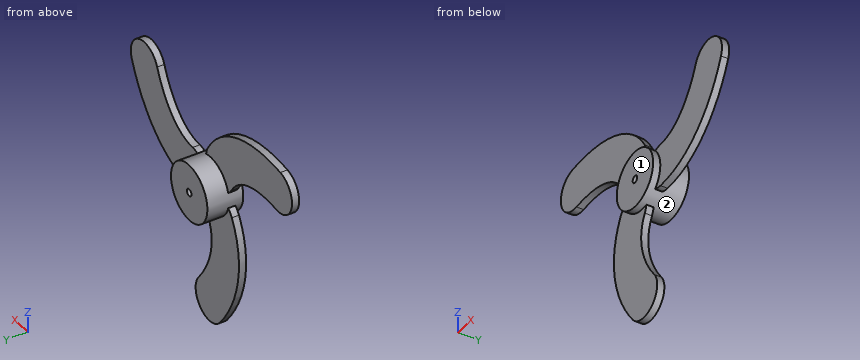
```python
from build123d import *

# Parameters (mm, degrees)
SKETCH1_R               = 4
BOSS_EXTRUDE1_DEPTH     = 5
BOSS_EXTRUDE2_START     = 1
BOSS_EXTRUDE2_DEPTH     = 1
SKETCH3_R               = 0.5
CUT_EXTRUDE1_DEPTH      = 1
CUT_EXTRUDE1_DEPTH_BACK = 6


with BuildPart() as part:
    # Sketch1 → Boss-Extrude1 (new body)
    with BuildSketch(Plane(origin=(0, 0, 0), x_dir=(1, 0, 0), z_dir=(0, 1, 0))):
        Circle(SKETCH1_R)
    extrude(amount=BOSS_EXTRUDE1_DEPTH)

    # Sketch2 → Boss-Extrude2 (add)
    with BuildSketch(Plane(origin=(0, 0, 0), x_dir=(1, 0, 0), z_dir=(0, 1, 0)).offset(BOSS_EXTRUDE2_START)):
        with BuildLine():
            ThreePointArc((3.96292251, -2.970932025), (3.419315306, -2.914444777), (2.894976906, -2.760273305))
            ThreePointArc((2.894976906, -2.760273305), (3.99989603, 0.028840126), (2.854873637, 2.801730986))
            ThreePointArc((2.854873637, 2.801730986), (3.434376926, 2.975056029), (4.036869549, 3.028612277))
            add(Edge.make_bspline(
                [(4.036869549, 3.028612277), (4.461696183, 3.023376101), (5.318698227, 2.968686223), (6.954159562, 2.692039011), (9.640789789, 1.796530328), (12.810078972, -0.41937164), (15.116309585, -3.289140753), (16.531628152, -5.76825703), (17.095168614, -7.020174314), (17.350686676, -7.663372062)],
                knots=[0, 0, 0, 0, 0.0625, 0.125, 0.25, 0.5, 0.75, 0.875, 1, 1, 1, 1], degree=3))
            ThreePointArc((17.350686676, -7.663372062), (15.67022042, -11.559014905), (11.774577577, -9.878548648))
            add(Edge.make_bspline(
                [(3.96292251, -2.970932025), (4.182230159, -2.973635089), (4.62835587, -3.002140243), (5.450410806, -3.141998702), (6.419949985, -3.462832618), (7.519073058, -4.074722518), (8.911985554, -5.187495456), (10.473170644, -7.100700539), (11.40121591, -8.938711436), (11.774577577, -9.878548648)],
                knots=[0, 0, 0, 0, 0.0625, 0.125, 0.25, 0.375, 0.5, 0.75, 1, 1, 1, 1], degree=3))
        make_face()
        with BuildLine():
            ThreePointArc((-3.837955256, -1.126986891), (-1.974971733, -3.478431637), (0.99893339, -3.873258587))
            ThreePointArc((0.99893339, -3.873258587), (0.859285635, -4.461785679), (0.604420396, -5.01033772))
            add(Edge.make_bspline(
                [(0.604420396, -5.01033772), (0.387472417, -5.375630289), (-0.088391429, -6.090470891), (-1.145705609, -7.368498348), (-3.264553992, -9.247434034), (-6.768225979, -10.884167994), (-10.406634241, -11.446537736), (-13.2612712, -11.432681431), (-14.627233602, -11.294763145), (-15.312018222, -11.194449404)],
                knots=[0, 0, 0, 0, 0.0625, 0.125, 0.25, 0.5, 0.75, 0.875, 1, 1, 1, 1], degree=3))
            ThreePointArc((-15.312018222, -11.194449404), (-17.84551076, -7.791301514), (-14.44236287, -5.257808976))
            add(Edge.make_bspline(
                [(-4.554363861, -1.946525554), (-4.666358608, -2.135100018), (-4.914107651, -2.507203639), (-5.446256097, -3.149194868), (-6.208876009, -3.828423469), (-7.288349743, -4.474347022), (-8.948495624, -5.12425816), (-11.385972373, -5.519681567), (-13.441759135, -5.404386894), (-14.44236287, -5.257808976)],
                knots=[0, 0, 0, 0, 0.0625, 0.125, 0.25, 0.375, 0.5, 0.75, 1, 1, 1, 1], degree=3))
            ThreePointArc((-4.554363861, -1.946525554), (-4.233640868, -1.50399153), (-3.837955256, -1.126986891))
        make_face()
        with BuildLine():
            ThreePointArc((0.94297835, 3.887260196), (-2.024924297, 3.449591511), (-3.853807027, 1.071527601))
            ThreePointArc((-3.853807027, 1.071527601), (-4.293662561, 1.48672965), (-4.641289945, 1.981725443))
            add(Edge.make_bspline(
                [(-4.641289945, 1.981725443), (-4.8491686, 2.352254188), (-5.230306799, 3.121784668), (-5.808453952, 4.676459337), (-6.376235797, 7.450903706), (-6.041852992, 11.303539634), (-4.709675344, 14.735678488), (-3.270356952, 17.200938461), (-2.467935012, 18.314937459), (-2.038668454, 18.857821466)],
                knots=[0, 0, 0, 0, 0.0625, 0.125, 0.25, 0.5, 0.75, 0.875, 1, 1, 1, 1], degree=3))
            ThreePointArc((-2.038668454, 18.857821466), (2.17529034, 19.350316419), (2.667785293, 15.136357624))
            add(Edge.make_bspline(
                [(0.591441352, 4.917457579), (0.484128449, 5.108735107), (0.285751781, 5.509343883), (-0.004154708, 6.29119357), (-0.211073976, 7.291256087), (-0.230723315, 8.54906954), (0.03651007, 10.311753616), (0.912801729, 12.620382105), (2.040543226, 14.34309833), (2.667785293, 15.136357624)],
                knots=[0, 0, 0, 0, 0.0625, 0.125, 0.25, 0.375, 0.5, 0.75, 1, 1, 1, 1], degree=3))
            ThreePointArc((0.591441352, 4.917457579), (0.814325562, 4.418436307), (0.94297835, 3.887260196))
        make_face()
    extrude(amount=BOSS_EXTRUDE2_DEPTH)

    # Sketch3 → Cut-Extrude1 (cut, two sides)
    with BuildSketch(Plane(origin=(0, 5, 0), x_dir=(1, 0, 0), z_dir=(0, 1, 0))) as cut_extrude1_sk:
        Circle(SKETCH3_R)
    extrude(amount=CUT_EXTRUDE1_DEPTH, mode=Mode.SUBTRACT)
    extrude(cut_extrude1_sk.sketch, amount=-CUT_EXTRUDE1_DEPTH_BACK, mode=Mode.SUBTRACT)


solid = part.part
```
Verification items for the finished model (mm, model axes). Face numbers are marked on the shaded views. A direction names the side the tool comes from. Give positions to 0.01 mm unless a question says otherwise; leave off trailing zeros. Order: outer loops, then holes, each group sorted by start corner. A loop starts at its lowest first (then second) coordinate and runs counter-clockwise, first axis right, second up. Notation, with made-up numbers: (51.25, -26) - (71.25, -26) arc R18 cw to (71.25, -14) - close; hole circle Ø6 at (-11, 29). An arc over 180 degrees is marked (long way). Answer as CSV lines item,"result". Start each with the question number.
Item 1: Access from +Z, -Z, +X, -X, +Y, -Y to the whole of each face (thin tool, end or side, straight path). Record for the marked faces 1 and 2.
Item 2: Gauge pin test, flat ends, axial feed: pin 1 (2 mm diameter, centred on x = 10, y = 2, fed in from +Z); pin 2 (1 mm diameter, centred on y = 3, z = -8, fed in from +X); pin 3 (7.5 mm diameter, centred on x = 0, z = -9.5, fed in from +Y); pin 4 (5 mm diameter, centred on x = -1.5, z = -13, fed in from -Y). Record the tip position at first contact, or that the pin passes through.
Item 3: Material ranges on L1, parallel to X at y = 2.6, z = 0; L2, parallel to Y at x = -11, z = 7, recorded low to high.
Item 4: Section check A-A, the plane y = 4.6. Record the boundary of the cut face in (x, z), plus the area to 3 significant figures.
Filled in:
1,face 1,"+Z, -Z, +X, -X, -Y"
1,face 2,"none"
2,pin 1,"z = 8.21"
2,pin 2,"through"
2,pin 3,"y = 2"
2,pin 4,"y = 1"
3,L1,"-4 to -0.5, 0.5 to 4"
3,L2,"1 to 2"
4,outline,"circle Ø8 at (0, 0); hole circle Ø1 at (0, 0)"
4,area,"49.5 mm^2"
